Geometry: final body of the model. Coordinates: model frame, mm. A direction names the side the tool comes from. Give positions to 0.01 mm unless a question says otherwise; leave off trailing zeros. Order: outer loops, then holes, each group sorted by start corner. A loop starts at its lowest first (then second) coordinate and runs counter-clockwise, first axis right, second up. Notation, with made-up numbers: (53.25, 63) - (90.25, 63) arc R32 ccw to (90.25, 96) - close; hole circle Ø6 at (-21.5, 12.25). An arc over 180 degrees is marked (long way). One line per item, written item: value.
Autodesk Inventor part; units mm, degrees
ref_plane "YZ Plane" through (0, 0, 0) normal (1, 0, 0) x (0, 1, 0)
ref_plane "XZ Plane" through (0, 0, 0) normal (0, 1, 0) x (-1, 0, 0)
ref_plane "XY Plane" through (0, 0, 0) normal (0, 0, 1) x (1, 0, 0)
sketch "スケッチ1" plane through (0, 0, 0) normal (0, 0, 1) x (1, 0, 0)
  line L0 (-45.5, -42) -> (45.5, -42)
  line L1 (45.5, -42) -> (45.5, 22)
  line L2 (45.5, 22) -> (-45.5, 22)
  line L3 (-45.5, 22) -> (-45.5, -42)
  line L4 (-45.5, 0) -> (0, 0)
  line L5 (0, 0) -> (45.5, 0)
  dimension "d0" = 64
  dimension "d1" = 91
  dimension "d20" = 42
extrude "外枠2" add sketch "スケッチ1" along normal blind 59
sketch "スケッチ２" plane through (0, 0, 0) normal (0, 0, -1) x (1, 0, 0)
  line L0 (43.5, -20) -> (-43.5, -20)
  line L1 (-43.5, -20) -> (-43.5, 20)
  line L2 (-43.5, 20) -> (43.5, 20)
  line L3 (43.5, 20) -> (43.5, -20)
  line L4 (43.5, -20) -> (-43.5, 20) construction
  line L5 (-43.5, -20) -> (43.5, 20) construction
  point P0 (0, 0)
  dimension "d4" = 40
  dimension "d5" = 87
extrude "本体" cut sketch "スケッチ２" against normal blind 59
sketch "スケッチ4" plane through (-45.5, 22, 0) normal (0, 1, 0) x (1, 0, 0)
  line L0 (0, -59) -> (91, -59)
  line L1 (0, 0) -> (91, 0)
  line L2 (91, -59) -> (0, -59)
  line L3 (0, -59) -> (0, 0)
  line L4 (0, 0) -> (91, 0)
  line L5 (91, 0) -> (91, -59)
  point P0 (45.5, 0)
extrude "上くり抜き" cut sketch "スケッチ4" against normal blind 2
sketch "スケッチ5" plane through (0, 0, 0) normal (0, 0, -1) x (-1, 0, 0)
  line L0 (-43.5, -20) -> (-43.5, 20)
  line L1 (-43.5, 20) -> (-38.5, 20)
  line L2 (-38.5, 20) -> (-38.5, -13)
  line L3 (-38.5, -13) -> (33.5, -13)
  line L4 (33.5, -13) -> (33.5, 20)
  line L5 (43.5, -20) -> (43.5, 20)
  line L6 (33.5, 20) -> (43.5, 20)
  line L7 (43.5, 20) -> (43.5, -20)
  line L8 (43.5, -20) -> (-43.5, -20)
  line L9 (43.5, -20) -> (-43.5, -20)
  line L10 (-43.5, -20) -> (-43.5, 20)
  point P0 (0, 0)
  dimension "d15" = 5
  dimension "d16" = 10
  dimension "d17" = 33
extrude "側面" add sketch "スケッチ5" against normal blind 2
sketch "スケッチ6" plane through (43.5, -20, 59) normal (-1, 0, 0) x (0, 0, 1)
  line L0 (-49, 5.5) -> (-29, 5.5)
  line L1 (-29, 5.5) -> (-29, 1.5)
  line L2 (-29, 1.5) -> (-49, 1.5)
  line L3 (-49, 1.5) -> (-49, 5.5)
  line L4 (-17, 5.5) -> (-7, 5.5)
  line L5 (-7, 5.5) -> (-7, 1.5)
  line L6 (-7, 1.5) -> (-17, 1.5)
  line L7 (-17, 1.5) -> (-17, 5.5)
  line L8 (-57, 0) -> (0, 0)
  line L9 (0, 40) -> (0, 0)
  point P0 (-59, 20)
  point P1 (-57, 7)
  dimension "d21" = 1.5
  dimension "d22" = 8
  dimension "d23" = 20
  dimension "d24" = 10
  dimension "d25" = 7
  dimension "d26" = 4
  dimension "d27" = 4
extrude "支え" add sketch "スケッチ6" along normal blind 15
sketch "スケッチ9" plane through (0, 0, 0) normal (0, 0, -1) x (-1, 0, 0)
  line L0 (-45.5, -42) -> (-45.5, 20)
  line L1 (-45.5, -25) -> (-30.5, -25)
  line L2 (-30.5, -25) -> (-30.5, -40)
  line L3 (-30.5, -40) -> (-45.5, -40)
  line L4 (-45.5, -40) -> (-45.5, -25)
  line L5 (45.5, 20) -> (45.5, -42)
  line L6 (45.5, -25) -> (30.5, -25)
  line L7 (30.5, -25) -> (30.5, -40)
  line L8 (30.5, -40) -> (45.5, -40)
  line L9 (45.5, -40) -> (45.5, -25)
  line L10 (45.5, -42) -> (-45.5, -42)
  point P0 (0, 0)
  dimension "d38" = 2
  dimension "d39" = 15
  dimension "d40" = 15
  dimension "d41" = 15
extrude "ネジ穴1" cut sketch "スケッチ9" against normal blind 15
sketch "スケッチ10" plane through (0, 0, 59) normal (0, 0, 1) x (1, 0, 0)
  line L0 (-45.5, -25) -> (-45.5, -40)
  line L1 (-45.5, -25) -> (-30.5, -25)
  line L2 (-30.5, -25) -> (-30.5, -40)
  line L3 (-30.5, -40) -> (-45.5, -40)
  line L4 (-45.5, -40) -> (-45.5, -25)
  line L5 (45.5, -40) -> (45.5, -25)
  line L6 (45.5, -25) -> (30.5, -25)
  line L7 (30.5, -25) -> (30.5, -40)
  line L8 (30.5, -40) -> (45.5, -40)
  line L9 (45.5, -40) -> (45.5, -25)
  line L10 (-45.5, -42) -> (45.5, -42)
  point P0 (0, 0)
  dimension "d44" = 15
  dimension "d45" = 2
  dimension "d46" = 2
  dimension "d47" = 15
  dimension "d48" = 15
  dimension "d49" = 15
extrude "ネジ穴2" cut sketch "スケッチ10" against normal blind 15
sketch "スケッチ15" plane through (-45.5, 20, 0) normal (0, 1, 0) x (1, 0, 0)
  line L0 (76, -59) -> (91, -59)
  line L1 (84, 0) -> (91, 0)
  line L2 (91, -59) -> (91, 0)
  line L3 (91, 0) -> (84, 0)
  line L4 (84, 0) -> (84, -2)
  line L5 (84, 0) -> (84, -2)
  line L6 (89, -2) -> (84, -2)
  line L7 (84, -2) -> (89, -2)
  line L8 (89, -2) -> (89, -59)
  line L9 (89, -2) -> (89, -59)
  line L10 (89, -59) -> (2, -59)
  line L11 (2, -2) -> (2, -59)
  line L12 (2, -59) -> (2, -2)
  line L13 (84, -2) -> (12, -2)
  line L14 (2, -2) -> (12, -2)
  line L15 (12, 0) -> (12, -2)
  line L16 (12, -2) -> (12, 0)
  line L17 (15, 0) -> (0, 0)
  line L18 (12, 0) -> (0, 0)
  line L19 (0, 0) -> (0, -59)
  line L20 (0, 0) -> (0, -59)
  line L21 (0, -59) -> (2, -59)
  point P0 (45.5, 0)
extrude "押し出し11" cut sketch "スケッチ15" against normal blind 30 contours L8 L6 L4 L1 L2 L0 | L21 L19 L17 L15 L14 L11
sketch "スケッチ17" plane through (-45.5, -42, 0) normal (0, -1, 0) x (1, 0, 0)
  line L0 (91, 59) -> (91, 44)
  line L1 (15, 0) -> (0, 0)
  line L2 (91, 0) -> (91, 59)
  line L3 (5.5, 3.5) -> (82.5, 3.5)
  line L4 (82.5, 3.5) -> (82.5, 55.5)
  line L5 (82.5, 55.5) -> (5.5, 55.5)
  line L6 (5.5, 55.5) -> (5.5, 3.5)
  line L7 (5.5, 3.5) -> (82.5, 55.5) construction
  line L8 (82.5, 3.5) -> (5.5, 55.5) construction
  point P0 (45.5, 0)
  point P1 (44, 29.5)
  dimension "d55" = 77
  dimension "d56" = 52
hole "穴1" at (-40, -42, 55.5) at (-40, -42, 3.5) at (37, -42, 55.5) at (37, -42, 3.5) direction (0, 1, 0) diameter 3 depth 2 tip angle 118
properties part number "ultra96_holder"
1) Section B-B, the plane z = 3.5. Return loops of the section in (x, y), then the cut area to 3 significant figures.
Answers below:
outline: (-45.5, -42) - (-41.5, -42) - (-41.5, -40) - (-45.5, -40) - close; (-45.5, -25) - (-30.5, -25) - (-30.5, -40) - (-38.5, -40) - (-38.5, -42) - (35.5, -42) - (35.5, -40) - (30.5, -40) - (30.5, -25) - (45.5, -25) - (45.5, -10) - (43.5, -10) - (43.5, -20) - (-43.5, -20) - (-43.5, -10) - (-45.5, -10) - close; (38.5, -42) - (45.5, -42) - (45.5, -40) - (38.5, -40) - close
area: 1,580 mm^2
2) Section D-D, the plane x = 37. Count the separate pieces of the cut face and the enclosed holes in it, then the cut area to 3 significant figures.
Answers below:
separate pieces: 5
enclosed holes: 0
area: 970 mm^2
3) Section A-A, the plane x = -40. Return loops of the section in (y, z), then the cut area to 3 significant figures.
Answers below:
outline: (-42, 0) - (-40, 0) - (-40, 2) - (-42, 2) - close; (-42, 5) - (-40, 5) - (-40, 15) - (-25, 15) - (-25, 0) - (-10, 0) - (-10, 2) - (-20, 2) - (-20, 59) - (-25, 59) - (-25, 44) - (-40, 44) - (-40, 54) - (-42, 54) - close; (-42, 57) - (-40, 57) - (-40, 59) - (-42, 59) - close
area: 856 mm^2
4) Set-up query: faces 1 (the face through (38, -25, 7)), 2 (the face through (36, -18.5, 20)), 3 (the face through (-38, -25, 7)), 4 (the face through (36, -17, 10)), 5 (the face through (30.5, -32, 52)). Return all of +Z, -Z, +X, -X, +Y, -Y with unobstructed straight access to the full face (end or side cutting, diameter ignored); none if empty.
Answers below:
face 1: -Z, +X
face 2: +Z
face 3: -Z, -X
face 4: +Y
face 5: +Z, +X
5) Material intervals for line 1 along Z through (x, y) = (37, -41); line 2 along X through (y, z) = (-40.75, 55.5); line 3 along Y through (x, z) = (-2, 22), sorted ascending.
Answers below:
line 1: 0 to 2, 5 to 54, 57 to 59
line 2: -45.5 to -41.5, -38.5 to 35.5, 38.5 to 45.5
line 3: -42 to -20
6) Section C-C, the plane y = -17. Return loops of the section in (x, z), then the cut area to 3 significant figures.
Answers below:
outline: (-45.5, 0) - (45.5, 0) - (45.5, 59) - (43.5, 59) - (43.5, 52) - (28.5, 52) - (28.5, 42) - (43.5, 42) - (43.5, 30) - (28.5, 30) - (28.5, 10) - (43.5, 10) - (43.5, 2) - (-43.5, 2) - (-43.5, 59) - (-45.5, 59) - close
area: 860 mm^2
7) Mould query, pull axis Y, two halves, no side actions, for faces 6 (the face through (38.33, -40.99, 54.81)), 7 (the face through (-44, -10, 25)), 8 (the face through (-38, -40, 7)), 9 (the face through (38, -40, 7)). Classes: released by +Y, released by -Y, zero draft, split by the parting line, or undercut.
Answers below:
face 6: zero draft
face 7: released by +Y
face 8: undercut
face 9: undercut
8) First-contact query: pin 1 (4.5 mm diameter, centred on x = 34.5, y = -36, fed in from -Z); pin 2 (7.5 mm diameter, centred on y = -34, z = 51.5, fed in from -X); pin 3 (10 mm diameter, centred on x = 21.5, z = 50, fed in from +Y). Flat tips, straight axial feed; report the tip coordinate or a pass-through.
Answers below:
pin 1: z = 15
pin 2: x = -30.5
pin 3: y = -20
